```python
from build123d import *

# Parameters (mm, degrees)
BOSS_EXTRUDE1_DEPTH = 6.35
SKETCH1_3_W         = 6.477
SKETCH1_3_H         = 6.35
BOSS_EXTRUDE2_DEPTH = 1.524
SKETCH2_R           = 1.5875
CUT_EXTRUDE1_DEPTH  = 51.8
FILLET1_R           = 4.826
FILLET2_R           = 6.35
SKETCH4_W           = 4.826
SKETCH4_H           = 33.0835
CUT_EXTRUDE5_DEPTH  = 47.625


with BuildPart() as part:
    # Sketch1 → Boss-Extrude1 (new body, symmetric)
    with BuildSketch(Plane(origin=(0, 0, 0), x_dir=(0, 0, -1), z_dir=(1, 0, 0))):
        Polygon((-19.939, 3.175), (-19.939, 0), (19.939, 0), (19.939, 50.8), (13.1445, 50.8), (13.1445, 35.729333418), (-5.167312548, 3.175), align=None)
    extrude(amount=BOSS_EXTRUDE1_DEPTH, both=True)

    # Sketch1<3> → Boss-Extrude2 (add, symmetric)
    with BuildSketch(Plane(origin=(0, 0, 0), x_dir=(0, 0, -1), z_dir=(1, 0, 0))):
        Polygon((13.1445, 0), (12.065, 0), (12.065, -6.35), (19.939, -6.35), (19.939, 0), align=None)
        with Locations((2.4765, -3.175)):
            Rectangle(SKETCH1_3_W, SKETCH1_3_H)
    extrude(amount=BOSS_EXTRUDE2_DEPTH, both=True)

    # Sketch2 → Cut-Extrude1 (cut, through all)
    with BuildSketch(Plane.XZ):
        with Locations((0, 15.1765)):
            Circle(SKETCH2_R)
    extrude(amount=-CUT_EXTRUDE1_DEPTH, mode=Mode.SUBTRACT)

    # Fillet1
    fillet1_edges = [part.edges().sort_by_distance(p)[0] for p in [
        (-6.35, 25.4, -19.939),
        (6.35, 25.4, -19.939),
    ]]
    fillet(fillet1_edges, radius=FILLET1_R)

    # Fillet2
    fillet2_edges = [part.edges().sort_by_distance(p)[0] for p in [
        (0, 3.175, 5.167312548),
    ]]
    fillet(fillet2_edges, radius=FILLET2_R)

    # Sketch4 → Cut-Extrude5 (cut)
    with BuildSketch(Plane(origin=(0, 50.8, 0), x_dir=(1, 0, 0), z_dir=(0, 1, 0))):
        with Locations((-3.937, -3.39725)):
            Rectangle(SKETCH4_W, SKETCH4_H)
        with Locations((3.937, -3.39725)):
            Rectangle(SKETCH4_W, SKETCH4_H)
    extrude(amount=-CUT_EXTRUDE5_DEPTH, mode=Mode.SUBTRACT)


solid = part.part
```
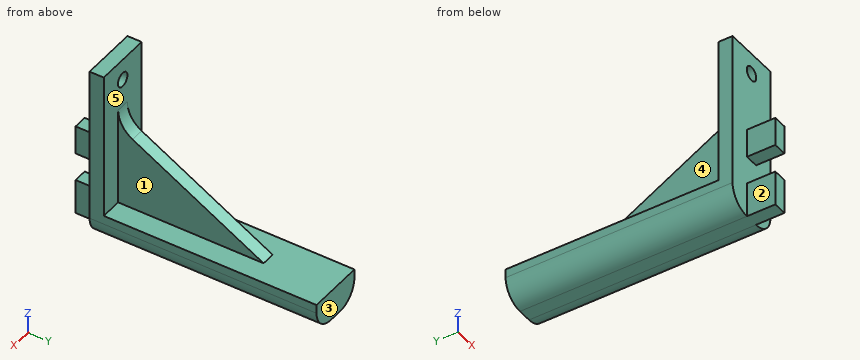
CAD build for the part. Positions are in the model's coordinates, mm. Face numbers are marked on the shaded views. A direction names the side the tool comes from. Coordinates: 2 decimals unless noted, no trailing zeros. Order: outer loops, then holes, each group sorted by start corner. A loop starts at its lowest first (then second) coordinate and runs counter-clockwise, first axis right, second up. Notation, with made-up numbers: (-18, 30.25) - (2, 30.25) arc R18 cw to (2, 36.25) - close; hole circle Ø10 at (-18, 74.5). An arc over 180 degrees is marked (long way). Answer in a Markdown table with one row per item.
1. Flat gauge pins, fed straight in: P1, Ø6.5, axis at x = -1.5, y = 23, coming from the +Z side; P2, Ø3, axis at x = -5, z = 12, coming from the +Y side (3 decimals); P3, Ø1.5, axis at x = 0.5, y = -4.5, coming from the +Z side. Where does each tip first touch, or does it go through?
Answer:
| item | result |
|---|---|
| P1 | z = -4.16 |
| P2 | y = 3.175 |
| P3 | z = 0.76 |
2. Drill centre lines: L1, parallel to Z at x = 0, y = 2.3; L2, parallel to Y at x = -4.5, z = 16.5 (3 decimals); L3, parallel to X at y = 4.5, z = -10. Where is each one in solid material? Low to high. Write a range as from..to.
Answer:
| item | result |
|---|---|
| L1 | -19.94..13.59, 16.76..19.94 |
| L2 | 0..3.175 |
| L3 | -1.52..1.52 |
3. Slice it at C-C, the plane x = -2.5. List the corners of the cut face in (y, z) (1 decimal).
Answer:
| item | result |
|---|---|
| outline | (0, -19.8) - (50.8, -19.8) - (50.8, -13.1) - (3.2, -13.1) - (3.2, 19.9) - (0, 19.9) - close |
4. Slice it at D-D, the plane z = 7. List the corners of the cut face in (x, y) (3 decimals).
Answer:
| item | result |
|---|---|
| outline | (-6.35, 0) - (6.35, 0) - (6.35, 3.175) - (1.524, 3.175) - (1.524, 3.46) - (-1.524, 3.46) - (-1.524, 3.175) - (-6.35, 3.175) - close |
5. 3-axis set-ups, long thin cutter, end or side, ignore diameter. For the marked faces 1, 2, 3, 4 and 5: which of +Z, -Z, +X, -X, +Y, -Y reach the whole face in a straight line?
Answer:
| item | result |
|---|---|
| face 1 | +Z, +X, +Y |
| face 2 | +Z, -Z, -X, -Y |
| face 3 | +Z, -Z, +X, -X, +Y |
| face 4 | +Z, -X, +Y |
| face 5 | +Z, +Y |
6. Slice it at B-B, the plane y = 45. List the corners of the cut face in (x, z), then the cut area to 3 significant figures.
Answer:
| item | result |
|---|---|
| outline | (-6.35, -15.11) arc R4.83 ccw to (-1.52, -19.94) - (1.52, -19.94) arc R4.83 ccw to (6.35, -15.11) - (6.35, -13.14) - (-6.35, -13.14) - close |
| area | 76.3 mm² |
